The model under review builds one solid part; all positions refer to its coordinate system, in mm. Face numbers are marked on the shaded views. A direction names the side the tool comes from. Give positions to 0.01 mm unless a question says otherwise; leave off trailing zeros. Order: outer loops, then holes, each group sorted by start corner. A loop starts at its lowest first (then second) coordinate and runs counter-clockwise, first axis right, second up. Notation, with made-up numbers: (16, -27) - (55, -27) arc R25 ccw to (55, 0) - close; hole circle Ø6 at (19, 72.5). An arc over 180 degrees is marked (long way). Use CSV: the item, a comma, the result in double quotes. Start each with the question number.
```python
from build123d import *

# Parameters (mm, degrees)
SKETCH1_W           = 48
SKETCH1_H           = 48
BOSS_EXTRUDE1_DEPTH = 9
SKETCH2_W           = 44
SKETCH2_H           = 44
CUT_EXTRUDE1_DEPTH  = 7
SKETCH3_R           = 6
BOSS_EXTRUDE2_DEPTH = 10
SKETCH4_R           = 3.6
CUT_EXTRUDE2_DEPTH  = 10
SKETCH5_W           = 30
SKETCH5_H           = 5
CUT_EXTRUDE3_DEPTH  = 10
FILLET1_R           = 2


with BuildPart() as part:
    # Sketch1 → Boss-Extrude1 (new body)
    with BuildSketch(Plane(origin=(0, 0, 0), x_dir=(1, 0, 0), z_dir=(0, 1, 0))):
        Rectangle(SKETCH1_W, SKETCH1_H)
    extrude(amount=BOSS_EXTRUDE1_DEPTH)

    # Sketch2 → Cut-Extrude1 (cut)
    with BuildSketch(Plane(origin=(0, 9, 0), x_dir=(1, 0, 0), z_dir=(0, 1, 0))):
        Rectangle(SKETCH2_W, SKETCH2_H)
    extrude(amount=-CUT_EXTRUDE1_DEPTH, mode=Mode.SUBTRACT)

    # Sketch3 → Boss-Extrude2 (add)
    with BuildSketch(Plane.XZ):
        with Locations(Location((0, 0, 0), (0, 0, 270))):
            Circle(SKETCH3_R)
    extrude(amount=BOSS_EXTRUDE2_DEPTH)

    # Sketch4 → Cut-Extrude2 (cut)
    with BuildSketch(Plane.XZ.offset(10)):
        with Locations(Location((0, 0, 0), (0, 0, 270))):
            Circle(SKETCH4_R)
    extrude(amount=-CUT_EXTRUDE2_DEPTH, mode=Mode.SUBTRACT)

    # Sketch5 → Cut-Extrude3 (cut)
    with BuildSketch(Plane.XY.offset(24)):
        with Locations((0, 4.5)):
            Rectangle(SKETCH5_W, SKETCH5_H)
    extrude(amount=-CUT_EXTRUDE3_DEPTH, mode=Mode.SUBTRACT)

    # Fillet1
    fillet1_edges = [part.edges().sort_by_distance(p)[0] for p in [
        (24, 4.5, 24),
        (-24, 4.5, 24),
        (-24, 4.5, -24),
        (24, 4.5, -24),
    ]]
    fillet(fillet1_edges, radius=FILLET1_R)


solid = part.part
```
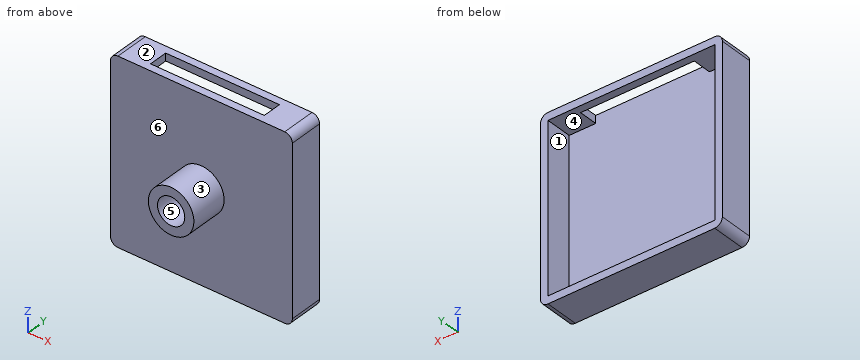
1. Consider section B-B (y = -6.25). Give the boundary of the cut face in (x, z), and give its area (3 significant figures).
2. Consider section A-A (x = -11.5). Give the boundary of the cut face in (y, z), and give its area (3 significant figures).
3. Tool access review of the marked faces 1 and 2: name each direction out of +Z, -Z, +X, -X, +Y, -Y from which nothing blocks a thin tool from reaching the whole face with its end or side.
4. Consider section C-C (z = 0). Give the boundary of the cut face in (x, y), and give its area (3 significant figures).
5. Mouldability with a two-part tool opening along X and no side actions: class the marked faces 3, 4, 5 and 6 as pulls with the +X half, pulls with the -X half, needs draft (parallel to the pull), parting line crosses it, or undercut.
6. To check wall thickness, follow L1, parallel to X at y = 8, z = 20; L2, parallel to X at y = -2.75, z = 0; L3, parallel to Y at x = 12, z = -4.5. State the ranges of each line that lie inside material, in increasing order. Write a range as [from, to].
7. Clearance check with flat-ended pins moving along their axes: pin 1 (10 mm diameter, centred on x = -4, z = 13, fed in from -Y); pin 2 (0.6 mm diameter, centred on y = 3.5, z = 23, fed in from -X); pin 3 (6 mm diameter, centred on x = 0, z = 0, fed in from +Y). State where each tip first meets the part, or that it passes through.
8. Consider section D-D (y = 6.25). Give the boundary of the cut face in (x, z), and give its area (3 significant figures).
Answers follow:
1,outline,"circle Ø12 at (0, 0); hole circle Ø7.2 at (0, 0)"
1,area,"72.4 mm^2"
2,outline,"(0, -24) - (9, -24) - (9, -22) - (2, -22) - (2, 24) - (0, 24) - close; (7, 22) - (9, 22) - (9, 24) - (7, 24) - close"
2,area,"114 mm^2"
3,face 1,"+Y"
3,face 2,"+Z, +X, -X, +Y, -Y"
4,outline,"(-24, 0) - (-6, 0) - (-6, -10) - (-3.6, -10) - (-3.6, 0) - (3.6, 0) - (3.6, -10) - (6, -10) - (6, 0) - (24, 0) - (24, 9) - (22, 9) - (22, 2) - (-22, 2) - (-22, 9) - (-24, 9) - close"
4,area,"172 mm^2"
5,face 3,"parting line crosses it"
5,face 4,"undercut"
5,face 5,"undercut"
5,face 6,"needs draft"
6,L1,"x = [-24, -22], [22, 24]"
6,L2,"x = [-6, -3.6], [3.6, 6]"
6,L3,"y = [0, 2]"
7,pin 1,"stops at y = 0"
7,pin 2,"stops at x = -23.87"
7,pin 3,"stops at y = 2"
8,outline,"(-24, -22) arc R2 ccw to (-22, -24) - (22, -24) arc R2 ccw to (24, -22) - (24, 22) arc R2 ccw to (22, 24) - (15, 24) - (15, 22) - (22, 22) - (22, -22) - (-22, -22) - (-22, 22) - (-15, 22) - (-15, 24) - (-22, 24) arc R2 ccw to (-24, 22) - close"
8,area,"305 mm^2"
